from build123d import *

# Parameters (mm, degrees)
RESSALTO_EXTRUS_O1_DEPTH = 30
ESBO_O2_R                = 1.5
CORTE_EXTRUS_O1_DEPTH    = 30
ESBO_O4_W                = 6.92820323
ESBO_O4_H                = 30
RESSALTO_EXTRUS_O2_DEPTH = 91
RESSALTO_EXTRUS_O3_DEPTH = 30


with BuildPart() as part:
    # Esboço1 → Ressalto-extrusão1 (new body)
    with BuildSketch(Plane(origin=(0, 0, 0), x_dir=(1, 0, 0), z_dir=(0, 1, 0))):
        Polygon((4.812291954, -4.984159523), (6.72255474, 1.675487321), (1.910262787, 6.659646844), (-4.812291954, 4.984159523), (-6.72255474, -1.675487321), (-1.910262787, -6.659646844), align=None)
    extrude(amount=RESSALTO_EXTRUS_O1_DEPTH)

    # Esboço2 → Corte-extrusão1 (cut)
    with BuildSketch(Plane.XZ):
        with Locations(Location((0, 0, 0), (0, 0, 270))):
            Circle(ESBO_O2_R)
    corte_extrus_o1 = extrude(amount=-CORTE_EXTRUS_O1_DEPTH, mode=Mode.SUBTRACT)

    # Esboço4 → Ressalto-extrusão2 (add)
    with BuildSketch(Plane(origin=(5.767423347, 0, 1.654336101), x_dir=(0.27572268356451307, 0, -0.961237224501831), z_dir=(0.961237224501831, 0, 0.27572268356451307))):
        with Locations((0, 15)):
            Rectangle(ESBO_O4_W, ESBO_O4_H)
    extrude(amount=RESSALTO_EXTRUS_O2_DEPTH)

    # Esboço5 → Ressalto-extrusão3 (add, through all)
    with BuildSketch(Plane(origin=(0, 0, 0), x_dir=(1, 0, 0), z_dir=(0, 1, 0))):
        Polygon((105.729988864, -26.723949087), (100.917696911, -21.739789563), (94.19514217, -23.415276884), (92.284879383, -30.074923728), (97.097171337, -35.059083251), (103.819726077, -33.38359593), align=None)
    extrude(amount=RESSALTO_EXTRUS_O3_DEPTH)

    # Espelhar1: Corte-extrusão1 across plane
    add(corte_extrus_o1.mirror(Plane(origin=(43.736293715, 0, 12.545382102), x_dir=(-0.2757226835645132, 0, 0.9612372245018309), z_dir=(-0.961237224501831, 0, -0.2757226835645132))), mode=Mode.SUBTRACT)


solid = part.part
Part model, mm, in its own coordinate system. A direction names the side the tool comes from. Round coordinates to 2 decimals unless told otherwise and drop trailing zeros. Write each loop counter-clockwise with the first axis right and the second up, starting at its lowest first coordinate (ties: lowest second). Pieces come first, ordered by that corner, then holes. Notation, with made-up numbers: (20, 17) - (29, 17) arc R16 ccw to (29, 40) - close; hole circle Ø9 at (31.5, -38). An arc over 180 degrees is marked (long way). Use CSV: the item, a comma, the result in double quotes.
Item 1: Slice it at D-D, the plane x = 79.5. Write the cut outline in (y, z).
Results list:
outline,"(0, 19.2) - (30, 19.2) - (30, 26.41) - (0, 26.41) - close"
Item 2: Tool access for faces 4 (the flat face through (1.404, 14.79, 5.834)), 5 (the flat face through (97.603, 14.79, 22.566)), 6 (the flat face through (-4.35, 14.79, 4.13)): list every direction of +Z, -Z, +X, -X, +Y, -Y with a clear straight run to the whole face (end or side of a thin tool).
Results list:
face 4,"+Z, +Y, -Y"
face 5,"-Z, +Y, -Y"
face 6,"+Z, -X, +Y, -Y"
Item 3: Slice it at C-C, the plane y = 18.5. Write the cut outline in (x, z).
Results list:
outline,"(-6.72, 1.68) - (-4.81, -4.98) - (1.91, -6.66) - (6.72, -1.68) - (94.2, 23.42) - (100.92, 21.74) - (105.73, 26.72) - (103.82, 33.38) - (97.1, 35.06) - (92.28, 30.07) - (4.81, 4.98) - (-1.91, 6.66) - close; hole circle Ø3 at (0, 0); hole circle Ø3 at (87.47, 25.09)"
Item 4: Wall check: L1, parallel to Z at x = 56.5, y = 11.5; L2, parallel to Z at x = 97, y = 9.25; L3, parallel to X at y = 24.25, z = -3. Give the ranges that are in metal, low to high.
Results list:
L1,"z = 12.6 to 19.81"
L2,"z = 22.72 to 34.96"
L3,"x = -5.38 to 5.44"
Item 5: Pull direction Z, two halves, no side cores. Call faces 1 (the flat face through (47.936, 14.79, 17.354)), 2 (the flat face through (4.35, 14.79, -4.13)), 3 (the cylindrical face through (87.616, 14.79, 26.584)): pulls with the +Z half, pulls with the -Z half, needs draft (parallel to the pull), parting line crosses it, or undercut.
Results list:
face 1,"pulls with the +Z half"
face 2,"pulls with the -Z half"
face 3,"undercut"
Item 6: Slice it at A-A, the plane x = 0. Write the cut outline in (y, z).
Results list:
outline,"(0, -6.18) - (30, -6.18) - (30, -1.5) - (0, -1.5) - close; (0, 1.5) - (30, 1.5) - (30, 6.18) - (0, 6.18) - close"
Item 7: Slice it at B-B, the plane z = 0. Write the cut outline in (x, y).
Results list:
outline,"(-6.24, 0) - (-1.5, 0) - (-1.5, 30) - (-6.24, 30) - close; (1.5, 0) - (12.56, 0) - (12.56, 30) - (1.5, 30) - close"
